Autodesk Inventor part; units mm, degrees
ref_plane "YZ Plane" through (0, 0, 0) normal (1, 0, 0) x (0, 1, 0)
ref_plane "XZ Plane" through (0, 0, 0) normal (0, 1, 0) x (-1, 0, 0)
ref_plane "XY Plane" through (0, 0, 0) normal (0, 0, 1) x (1, 0, 0)
sketch "Boceto1" plane through (0, 0, 0) normal (0, 1, 0) x (-1, 0, 0)
  line L0 (10.3005, 0.2018) -> (-1.6995, 0.2018)
  line L1 (-1.6995, 0.2018) -> (-1.6995, 18.2018)
  line L2 (-1.6995, 18.2018) -> (10.3005, 18.2018)
  line L3 (12.3005, 20.2018) -> (-3.6995, 20.2018)
  line L4 (-3.6995, 20.2018) -> (-3.6995, -1.7982)
  line L5 (-3.6995, -1.7982) -> (12.3005, -1.7982)
  line L6 (10.3005, 18.2018) -> (12.3005, 18.2018)
  line L7 (10.3005, 0.2018) -> (12.3005, 0.2018)
  line L8 (12.3005, -1.7982) -> (12.3005, 0.2018)
  line L9 (12.3005, 18.2018) -> (12.3005, 20.2018)
  point P0 (0, 0)
  point P1 (0, 0)
  dimension "d0" = 18
  dimension "d1" = 12
extrude "Extrusión1" add sketch "Boceto1" along normal blind 28
sketch "Boceto4" plane through (1.6995, 0, 0.2018) normal (-1, 0, 0) x (0, 0, 1)
  line L0 (18, 0) -> (18, 28)
  line L1 (18, 28) -> (18, 12)
  line L2 (18, 12) -> (0, 12)
  line L3 (0, 0) -> (0, 28)
  line L4 (18, 28) -> (0, 28)
  line L5 (0, 28) -> (0, 12)
  line L6 (20, 28) -> (-2, 28)
  line L7 (9, 28) -> (9, 12)
  circle A0 centre (9, 24) radius 1.75
  circle A1 centre (9, 16) radius 1.75
  line L8 (18, 12) -> (18, 0)
  line L9 (0, 0) -> (18, 0)
  line L10 (0, 0) -> (0, 12)
  line L11 (18, 0) -> (0, 0)
  point P0 (-0.2018, 0)
  dimension "d14" = 16
  dimension "d15" = 3.5
  dimension "d16" = 3.5
  dimension "d17" = 4
  dimension "d18" = 4
extrude "Extrusión4" cut sketch "Boceto4" against normal blind 2 contours L9 L3 L2 L0 | A1 L7 | L7 A1 | A0 L7 | L7 A0
sketch "Boceto5" plane through (3.6995, 28, -1.7982) normal (0, 0, -1) x (-1, 0, 0)
  line L0 (0, -28) -> (0, 0)
  line L1 (0, 0) -> (4, 0)
  line L2 (16, 0) -> (0, 0)
  line L3 (0, 0) -> (0, -16)
  line L4 (0, -16) -> (16, -16)
  line L5 (16, -28) -> (16, 0)
  line L6 (4, 0) -> (16, -16)
  line L7 (4, 0) -> (4, -16)
  point P0 (3.6995, -28)
  point P1 (0, -26.5)
  point P2 (16, -26.5)
  dimension "d21" = 4
  dimension "d22" = 16
extrude "Extrusión5" cut sketch "Boceto5" against normal blind 30 contours L2 L5 L6
sketch "Boceto6" plane through (3.6995, 0, -1.7982) normal (0, 0, -1) x (-1, 0, 0)
  line L0 (0, 12) -> (0, 0)
  line L1 (16, 0) -> (16, 12)
  arc A0 (0, 0) -> (16, 0) centre (8, -0.0553) ccw
  line L2 (16, 0) -> (0, 0)
  line L3 (16, 0) -> (0, 0)
  point P0 (3.6995, 0)
sketch "Boceto7" plane through (-12.3005, 0, 20.2018) normal (0, 0, 1) x (1, 0, 0)
  line L0 (0, 12) -> (0, 0)
  line L1 (16, 0) -> (16, 12)
  arc A0 (0, 0) -> (16, 0) centre (8, -0.0553) ccw
  line L2 (0, 0) -> (16, 0)
  line L3 (0, 0) -> (16, 0)
  circle A1 centre (8, -2.0553) radius 1.75
  point P0 (12.3005, 0)
  point P1 (3.6995, 0)
  dimension "d30" = 3.5
  dimension "d31" = 2
extrude "Extrusión6" add sketch "Boceto7" against normal blind 2 contours L2 A0 | A1
extrude "Extrusión7" add sketch "Boceto6" against normal blind 2
extrude "Extrusión8" cut sketch "Boceto7" against normal blind 30 contours A1
properties part number "Kit de Sujeción 2"
Here's how the part is built. I have some questions about the finished solid (model axes, mm). A direction names the side the tool comes from. Give positions to 0.01 mm unless a question says otherwise; leave off trailing zeros. Write each loop counter-clockwise with the first axis right and the second up, starting at its lowest first coordinate (ties: lowest second). Pieces come first, ordered by that corner, then holes. Notation, with made-up numbers: M 53.25,23.25 L 65.25,23.25 A23 cw 65.25,52.25 Z; hole C -18.75,-9.5 d7. An arc over 180 degrees is marked long. Put each result on its own line as item: value. Start each with the question number.
Item 1: Will these pins go through, and if not, where does the flat tip stop? pin 1 (8 mm diameter, centred on x = -1.5, z = 3.5, fed in from -Y); pin 2 (2 mm diameter, centred on y = 23.5, z = 3, fed in from -X); pin 3 (0.6 mm diameter, centred on x = 3, z = 7.5, fed in from -Y).
Item 2: If we section it at B-B, the plane x = -5.25: Write out the boundary of the cut face in (y, z), then the cut area to 3 significant figures.
Item 3: Thinking about a two-plate mould opening in X: for faces 4 (the cylindrical face through (-6.05, -1.98, 19.22)), 5 (the cylindrical face through (2.686, 25.735, 8.974)), 6 (the flat face through (3.7, 20, 9)), 7 (the flat face through (-6.22, 20.11, -0.81)), which applies, +X half, -X half, draft (parallel to the pull), parting line (faces both ways), or undercut?
Item 4: On a 3-axis mill with a long thin cutter (end or side, diameter ignored), from which of +Z, -Z, +X, -X, +Y, -Y can I reach the whole of each face in a straight line? I mean faces 1 (the cylindrical face through (2.686, 17.735, 8.974)), 2 (the flat face through (1.7, 20, 9)), 3 (the flat face through (3, 12, 9)). Say none if no direction works.
Item 5: If we section it at A-A, the plane y = 16: Write out the boundary of the cut face in (x, z).
Item 6: If we section it at D-D, the plane y = 8: Write out the boundary of the cut face in (x, z), then the cut area to 3 significant figures.
Item 7: If we section it at C-C, the plane x = -7.5: Write out the boundary of the cut face in (y, z), then the cut area to 3 significant figures.
Item 8: I need wall thicknesses on L1, parallel to Z at x = 2.5, y = 7; L2, parallel to Z at x = 3.25, y = 25.5; L3, parallel to X at y = 14, z = 17.25. Which ranges of each line are inside material? Lowest first, please. Write a range as from..to.
Values:
1. pin 1: y = -8.04
1. pin 2: x = 1.7
1. pin 3: y = 12
2. outline: M -8,-1.8 L -3.53,-1.8 L -3.53,0.2 L -8,0.2 Z; M -8,18.2 L -3.53,18.2 L -3.53,20.2 L -8,20.2 Z; M -0.59,-1.8 L 21.4,-1.8 L 21.4,0.2 L -0.59,0.2 Z; M -0.59,18.2 L 21.4,18.2 L 21.4,20.2 L -0.59,20.2 Z
2. area: 106 mm²
3. face 4: undercut
3. face 5: draft
3. face 6: +X half
3. face 7: -X half
4. face 1: +X, -X
4. face 2: -X, +Y, -Y
4. face 3: +X, -X, -Y
5. outline: M -9.3,-1.8 L 3.7,-1.8 L 3.7,7.45 L 1.7,7.45 L 1.7,0.2 L -9.3,0.2 Z; M -9.3,18.2 L 1.7,18.2 L 1.7,10.95 L 3.7,10.95 L 3.7,20.2 L -9.3,20.2 Z
6. outline: M -12.3,-1.8 L 3.7,-1.8 L 3.7,0.2 L -12.3,0.2 Z; M -12.3,18.2 L 3.7,18.2 L 3.7,20.2 L -12.3,20.2 Z
6. area: 64.0 mm²
7. outline: M -7.39,-1.8 L 18.4,-1.8 L 18.4,0.2 L -7.39,0.2 Z; M -7.39,18.2 L 18.4,18.2 L 18.4,20.2 L -7.39,20.2 Z
7. area: 103 mm²
8. L1: -1.8..0.2, 18.2..20.2
8. L2: -1.8..8.3, 10.1..20.2
8. L3: 1.7..3.7
